Work out the finished part from the listing and answer in its coordinate system (mm). Give positions to 0.01 mm unless a question says otherwise; leave off trailing zeros. Loops run counter-clockwise (first coordinate to the right, second up) from the corner with the lowest first, then second, coordinate; pieces in that order, holes last. Notation, with made-up numbers: (58, 30.25) - (101, 30.25) arc R21 cw to (101, 69.25) - close; hole circle Ø3 at (19, 48). An arc over 180 degrees is marked (long way). Use CSV: the item, a comma, the result in double quotes.
from build123d import *

# Parameters (mm, degrees)
BOSS_EXTRUDE1_DEPTH = 2.9718
CUT_EXTRUDE1_DEPTH  = 83.929967317


with BuildPart() as part:
    # Sketch1 → Boss-Extrude1 (new body)
    with BuildSketch(Plane.YZ):
        Polygon((-10.081561306, 16.077656644), (-6.906561306, 16.077656644), (-6.906561306, 25.616432341), (75.643438694, 25.616432341), (75.643438694, 16.077656644), (78.818438694, 16.077656644), (78.818438694, 9.72759764), (75.643438694, 9.72759764), (75.643438694, 0.216196324), (-6.906561306, 0.216196324), (-6.906561306, 9.72759764), (-10.081561306, 9.72759764), align=None)
    extrude(amount=BOSS_EXTRUDE1_DEPTH)

    # Sketch2 → Cut-Extrude1 (cut, through all)
    with BuildSketch(Plane.YZ.offset(2.9718)):
        Polygon((0.078438694, 25.616432341), (1.348438694, 25.616432341), (1.348438694, 23.076432341), (2.618438694, 23.076432341), (2.618438694, 21.806432341), (0.078438694, 21.806432341), align=None)
        Polygon((6.428438694, 23.076432341), (6.428438694, 21.806432341), (8.968438694, 21.806432341), (8.968438694, 25.616432341), (7.698438694, 25.616432341), (7.698438694, 23.076432341), align=None)
        Polygon((29.923438694, 25.616432341), (31.193438694, 25.616432341), (31.193438694, 23.076432341), (32.463438694, 23.076432341), (32.463438694, 21.806432341), (29.923438694, 21.806432341), align=None)
        Polygon((36.273438694, 23.076432341), (36.273438694, 21.806432341), (38.813438694, 21.806432341), (38.813438694, 25.616432341), (37.543438694, 25.616432341), (37.543438694, 23.076432341), align=None)
        Polygon((59.768438694, 25.616432341), (61.038438694, 25.616432341), (61.038438694, 23.076432341), (62.308438694, 23.076432341), (62.308438694, 21.806432341), (59.768438694, 21.806432341), align=None)
        Polygon((66.118438694, 23.076432341), (66.118438694, 21.806432341), (68.658438694, 21.806432341), (68.658438694, 25.616432341), (67.388438694, 25.616432341), (67.388438694, 23.076432341), align=None)
    extrude(amount=-CUT_EXTRUDE1_DEPTH, mode=Mode.SUBTRACT)


solid = part.part
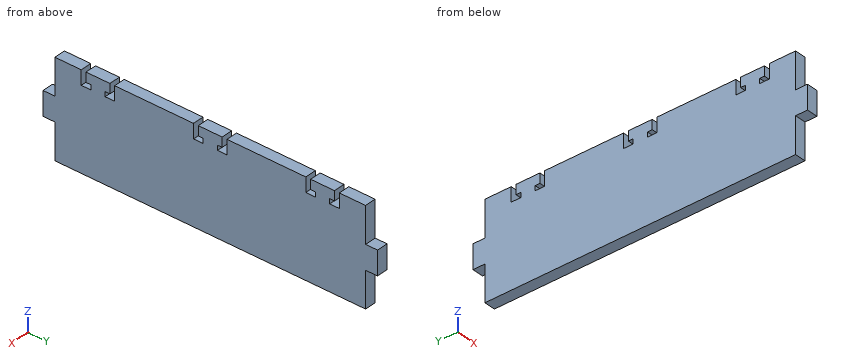
Item 1: Find the intervals of material crossed by line 1 (Z direction, x = 1.15, y = 61.5); line 2 (Y direction, x = 1.3, z = 20); line 3 (Z direction, x = 1.05, y = 60), in increasing order.
Determined:
line 1,"z = 0.22 to 21.81, 23.08 to 25.62"
line 2,"y = -6.91 to 75.64"
line 3,"z = 0.22 to 21.81"
Item 2: A cutting plane is placed at A-A on z = 5.25. Determine the outline of the cut face in (x, y).
Determined:
outline,"(0, -6.91) - (2.97, -6.91) - (2.97, 75.64) - (0, 75.64) - close"
Item 3: Given P1, Ø0.9, axis at x = 1, y = 77.5, coming from the +Z side; P2, Ø8, axis at y = 30.5, z = 19.5, coming from the -X side; P3, Ø1, axis at x = 2.5, z = 6, coming from the -Y side, each flat-ended and moving along its own axis, determine where each tip first touches the part or whether it passes through.
Determined:
P1,"stops at z = 16.08"
P2,"stops at x = 0"
P3,"stops at y = -6.91"
